```python
from build123d import *

# Parameters (mm, degrees)
F0_W     = 20
F0_H     = 20
F2_DEPTH = 25
F1_W     = 14.1000001311
F1_H     = 39.2423100663
F3_DEPTH = 25
F6_W     = 8.1000001311
F6_H     = 19
F7_DEPTH = 33.6010025272


with BuildPart() as f2:
    # F0 (on Front) → F2 (new body)
    with BuildSketch(Plane.XZ):
        with Locations((-1.2000007555, 1.4076924609)):
            Rectangle(F0_W, F0_H)
    extrude(amount=F2_DEPTH)

    # F1 (on Front) → F3 (join)
    with BuildSketch(Plane.XZ):
        with Locations((-1.2000008211, 13.9788474941)):
            Rectangle(F1_W, F1_H)
    extrude(amount=F3_DEPTH)

    # F5: sweep along a path in F5_path
    with BuildLine(Plane(origin=(-11.2000007555, 0, 11.4076924609), x_dir=(0, 1, 0), z_dir=(0, 0, 1))) as f5_path:
        Line((0, 0), (-25, 0))
    # F4 (on Front) → F5 (sweep)
    with BuildSketch(Plane.XZ):
        with BuildLine():
            ThreePointArc((0, -25.9104435142), (10.111753936, -21.7220178946), (14.3001795556, -11.6102639586))
            ThreePointArc((14.3001795556, -11.6102639586), (-10.111753936, -1.4985100226), (0, -25.9104435142))
        make_face()
    sweep(path=f5_path.line)

    # F6 (on Top) → F7 (cut, through all)
    with BuildSketch(Plane.XY):
        with Locations((-1.2000008211, -12.5)):
            Rectangle(F6_W, F6_H)
    extrude(amount=F7_DEPTH, mode=Mode.SUBTRACT)


solid = f2.part
```
Verification items for the finished model (mm, model axes). A direction names the side the tool comes from. Round coordinates to 2 decimals unless told otherwise and drop trailing zeros. Write each loop counter-clockwise with the first axis right and the second up, starting at its lowest first coordinate (ties: lowest second). Pieces come first, ordered by that corner, then holes. Notation, with made-up numbers: (12.25, 81.25) - (18.25, 81.25) arc R27 cw to (18.25, 98.25) - close; hole circle Ø7 at (-35.75, 48.5). An arc over 180 degrees is marked (long way). Answer as a JSON object with one key per item and string values. Group by question number.
Q1. Tool access check on faces 1 (the flat face through (-8.25, -12, 22)), 2 (the flat face through (7, -12, 11.408)), 3 (the flat face through (-1, -3, 17)), 4 (the flat face through (3, -12, 33.6)), 5 (the flat face through (0, 0, -2)). Record the directions out of +Z, -Z, +X, -X, +Y, -Y that give a thin tool (end or side, any length) a straight path to the whole face; none if there is none.
Q2. Section check D-D, the plane x = -2.25. Enter the section's corners in (y, z).
Q3. Section check A-A, the plane z = 28.5. Enter the section's corners in (x, y).
Q4. Mould release check, pull along X, two halves, no side actions. Record for faces 6 (the flat face through (0, -25, -2)), 7 (the flat face through (5.85, -12, 22)), 8 (the flat face through (-1, -22, 17)): released by +X, released by -X, zero draft, split by the parting line, or undercut.
Q5. Go/stop test with flat-tipped pins: pin 1 Ø1 at (y, z) = (-7.5, 16.5) entering from +X; pin 2 Ø4 at (x, y) = (-11, -12) entering from -Z; pin 3 Ø8 at (y, z) = (-19.5, 5.5) entering from -X. Record where each tip stops, or that it passes through.
Q6. Section check C-C, the plane z = 5.5. Enter the section's corners in (x, y), plus the area to 3 significant figures.
Q7. Thickness scan on line 1 (Y direction, x = -1.25, z = 26); line 2 (X direction, y = -20.25, z = 23); line 3 (X direction, y = -3.75, z = 5). Record the ranges inside material, lowest first.
Q8. Section check B-B, the plane y = -6.25. Enter the section's corners in (x, z).
Found:
{
 "1": {"face 1": "+Z, -X, +Y, -Y", "face 2": "+Z, +X, +Y, -Y", "face 3": "+Z", "face 4": "+Z, +X, -X, +Y, -Y", "face 5": "+Z, -Z, +X, -X, +Y"},
 "2": {"outline": "(-25, -25.73) - (0, -25.73) - (0, 33.6) - (-3, 33.6) - (-3, 0) - (-22, 0) - (-22, 33.6) - (-25, 33.6) - close"},
 "3": {"outline": "(-8.25, -25) - (5.85, -25) - (5.85, 0) - (-8.25, 0) - close; hole (-5.25, -22) - (2.85, -22) - (2.85, -3) - (-5.25, -3) - close"},
 "4": {"face 6": "zero draft", "face 7": "released by +X", "face 8": "undercut"},
 "5": {"pin 1": "stops at x = 5.85", "pin 2": "stops at z = -22.72", "pin 3": "stops at x = -11.2"},
 "6": {"outline": "(-11.2, -25) - (8.8, -25) - (8.8, 0) - (-11.2, 0) - close; hole (-5.25, -22) - (2.85, -22) - (2.85, -3) - (-5.25, -3) - close", "area": "346 mm^2"},
 "7": {"line 1": "y = -25 to -22, -3 to 0", "line 2": "x = -8.25 to -5.25, 2.85 to 5.85", "line 3": "x = -11.2 to -5.25, 2.85 to 8.8"},
 "8": {"outline": "(-11.2, -2.72) arc R14.3 ccw (long way) to (8.8, -0.34) - (8.8, 11.41) - (5.85, 11.41) - (5.85, 33.6) - (2.85, 33.6) - (2.85, 0) - (-5.25, 0) - (-5.25, 33.6) - (-8.25, 33.6) - (-8.25, 11.41) - (-11.2, 11.41) - close"}
}
